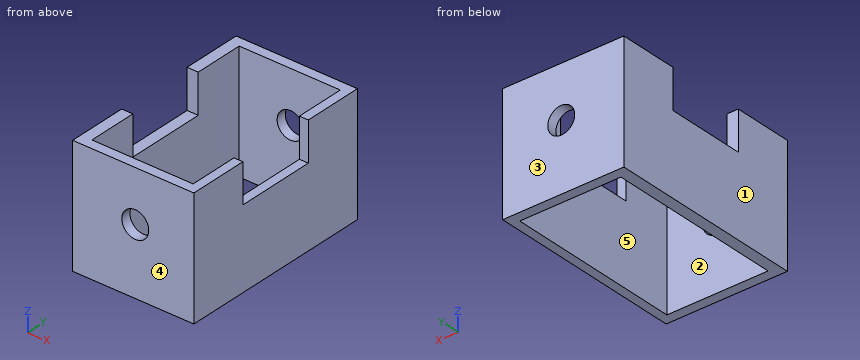
from build123d import *

# Parameters (mm, degrees)
F0_W     = 77.707555145
F0_H     = 127
F1_DEPTH = 76.2
F2_W     = 64.8572534889
F2_H     = 114.3
F3_DEPTH = 123.444
F4_R     = 8.6449584046
F5_DEPTH = 116.078
F6_W     = 50.8
F6_H     = 25.32691136
F7_DEPTH = 58.674


with BuildPart() as f1:
    # F0 (on Top) → F1 (new body)
    with BuildSketch(Plane.XY):
        with Locations((-1.2951251119, 0)):
            Rectangle(F0_W, F0_H)
    extrude(amount=F1_DEPTH)

    # F2 (on Top) → F3 (cut)
    with BuildSketch(Plane.XY):
        with Locations((-0.5756113678, 0)):
            Rectangle(F2_W, F2_H)
    extrude(amount=F3_DEPTH, mode=Mode.SUBTRACT)

    # F4 (on Front) → F5 (cut, symmetric)
    with BuildSketch(Plane.XZ):
        with Locations((0, 43.0269613862)):
            Circle(F4_R)
    extrude(amount=F5_DEPTH, both=True, mode=Mode.SUBTRACT)

    # F6 (on Right) → F7 (cut, symmetric)
    with BuildSketch(Plane.YZ):
        with Locations((0, 63.7489762157)):
            Rectangle(F6_W, F6_H)
    extrude(amount=F7_DEPTH, both=True, mode=Mode.SUBTRACT)


solid = f1.part
Verification items for the finished model (mm, model axes). Face numbers are marked on the shaded views. A direction names the side the tool comes from. Round coordinates to 2 decimals unless told otherwise and drop trailing zeros. Loops run counter-clockwise (first coordinate to the right, second up) from the corner with the lowest first, then second, coordinate; pieces in that order, holes last. Notation, with made-up numbers: (33, 42.5) - (73, 42.5) arc R33 cw to (73, 79.5) - close; hole circle Ø2 at (-6, -3.75). An arc over 180 degrees is marked (long way). Answer in a Markdown table with one row per item. Add a question column.
Q1. Release check for a two-part mould opening along Y. For the marked faces 3, 4 and 5 record: pulls with the +Y half, pulls with the -Y half, needs draft (parallel to the pull), parting line crosses it, or undercut.
Q2. Gauge pin test, flat end, axial feed: pin 1 (2 mm diameter, centred on x = -35.5, y = -8, fed in from +Z). Record the tip position at first contact, or that the pin passes through.
Q3. Material ranges on line 1 (Y direction, x = -19, z = 52); line 2 (Z direction, x = 0, y = 60.5); line 3 (X direction, y = -9.5, z = 33.5), recorded low to high.
Q4. Section check B-B on z = 8. Enter the section's corners in (x, y).
Q5. Section check A-A on y = -16. Enter the section's corners in (x, z), plus the area to 3 significant figures.
Q6. Tool access check on the marked faces 1 and 2. Record the directions out of +Z, -Z, +X, -X, +Y, -Y that give a thin tool (end or side, any length) a straight path to the whole face; none if there is none.
Q7. Section check C-C on x = -1.5. Enter the section's corners in (y, z).
Q8. Section check D-D on z = 56.5. Enter the section's corners in (x, y).
Found:
| question | item | result |
|---|---|---|
| 1 | face 3 | pulls with the +Y half |
| 1 | face 4 | pulls with the -Y half |
| 1 | face 5 | undercut |
| 2 | pin 1 | stops at z = 51.09 |
| 3 | line 1 | y = -63.5 to -57.15, 57.15 to 63.5 |
| 3 | line 2 | z = 0 to 34.38, 51.67 to 76.2 |
| 3 | line 3 | x = -40.15 to -33, 31.85 to 37.56 |
| 4 | outline | (-40.15, -63.5) - (37.56, -63.5) - (37.56, 63.5) - (-40.15, 63.5) - close; hole (-33, -57.15) - (31.85, -57.15) - (31.85, 57.15) - (-33, 57.15) - close |
| 5 | outline | (-40.15, 0) - (-33, 0) - (-33, 51.09) - (-40.15, 51.09) - close; (31.85, 0) - (37.56, 0) - (37.56, 51.09) - (31.85, 51.09) - close |
| 5 | area | 656 mm² |
| 6 | face 1 | +Z, -Z, -X, +Y, -Y |
| 6 | face 2 | +Z, -Z |
| 7 | outline | (-63.5, 0) - (-57.15, 0) - (-57.15, 34.51) - (-63.5, 34.51) - close; (-63.5, 51.54) - (-57.15, 51.54) - (-57.15, 76.2) - (-63.5, 76.2) - close; (57.15, 0) - (63.5, 0) - (63.5, 34.51) - (57.15, 34.51) - close; (57.15, 51.54) - (63.5, 51.54) - (63.5, 76.2) - (57.15, 76.2) - close |
| 8 | outline | (-40.15, -63.5) - (37.56, -63.5) - (37.56, -25.4) - (31.85, -25.4) - (31.85, -57.15) - (-33, -57.15) - (-33, -25.4) - (-40.15, -25.4) - close; (-40.15, 25.4) - (-33, 25.4) - (-33, 57.15) - (31.85, 57.15) - (31.85, 25.4) - (37.56, 25.4) - (37.56, 63.5) - (-40.15, 63.5) - close |
